```python
from build123d import *

# Parameters (mm, degrees)
SKETCH1_W           = 53
SKETCH1_H           = 53
BOSS_EXTRUDE1_DEPTH = 14.5
BOSS_EXTRUDE2_DEPTH = 53
SKETCH5_R           = 68.311173766
CUT_EXTRUDE1_DEPTH  = 60
SCALE1_SCALE        = 4


with BuildPart() as part:
    # Sketch1 → Boss-Extrude1 (new body)
    with BuildSketch(Plane(origin=(0, 0, 0), x_dir=(0, 0, -1), z_dir=(1, 0, 0))):
        with Locations((-26.5, -26.5)):
            Rectangle(SKETCH1_W, SKETCH1_H)
    extrude(amount=BOSS_EXTRUDE1_DEPTH)

    # Sketch2 → Boss-Extrude2 (add)
    with BuildSketch(Plane.XZ.offset(53)):
        Polygon((0, 53), (-15.864497794, 64.526232333), (-15.864497794, -11.526232333), (0, 0), align=None)
    extrude(amount=-BOSS_EXTRUDE2_DEPTH)

    # Sketch5 → Cut-Extrude1 (cut)
    with BuildSketch(Plane(origin=(0, 0, 0), x_dir=(1, 0, 0), z_dir=(0, 1, 0))):
        with Locations((-74.352498141, -26.670023257)):
            Circle(SKETCH5_R)
    extrude(amount=-CUT_EXTRUDE1_DEPTH, mode=Mode.SUBTRACT)


with BuildPart() as part_1:
    # Scale1: scaled about (0, 0, 0)
    add(part.part.scale(SCALE1_SCALE))


solid = part_1.part
```
Here's how the part is built. I have some questions about the finished solid (model axes, mm). A direction names the side the tool comes from. Round coordinates to 2 decimals unless told otherwise and drop trailing zeros. Write each loop counter-clockwise with the first axis right and the second up, starting at its lowest first coordinate (ties: lowest second). Pieces come first, ordered by that corner, then holes.
Q1. Please list where these lines run through material, in increasing order: probe 1 along Z at (x, y) = (53.5, -122.5); probe 2 along Z at (x, y) = (-53, -155); probe 3 along X at (y, z) = (-73.5, 75.5).
Q2. If we section it at B-B on y = -125: Write out the boundary of the cut face in (x, z), plus the area to 3 significant figures.
Q3. Will these pins go through, and if not, where does the flat tip stop? P1, Ø10, axis at y = -47.5, z = 176.5, coming from the -X side; P2, Ø4, axis at x = 22, y = -52, coming from the +Z side; P3, Ø8, axis at x = 43, y = -82.5, coming from the -Z side.
Q4. Which directions (+Z, -Z, +X, -X, +Y, -Y) give clear straight access to the entire face, cutting with the end or side of a thin tool? Please do faces 5 (the flat face through (29, -107, 0)), 6 (the flat face through (-63.458, -107, -40)).
Q5. If we section it at A-A on x = -32: Write out the boundary of the cut face in (y, z).
Q6. If we section it at C-C on x = 32.5: Write out the boundary of the cut face in (y, z).
Q7. If we mould it in two halves opening along Z, with no side actions, what happens to faces 1 (the flat face through (29, -107, 212)), 2 (the flat face through (10, 0, 108)), 3 (the flat face through (-32.173, -107.484, -23.375)), 4 (the cylindrical face through (-24.173, -104.516, 108.757))? For each: +Z half, -Z half, draft (parallel to the pull), parting line (faces both ways), or undercut.
Q8. If we section it at D-D on z = 229.5: Write out the boundary of the cut face in (x, y), plus the area to 3 significant figures.
Answer below:
1. probe 1: z = 0 to 212
1. probe 2: z = -38.51 to -15.49, 228.85 to 250.51
1. probe 3: x = -25.95 to 58
2. outline: (-63.46, -46.1) - (0, 0) - (58, 0) - (58, 212) - (0, 212) - (-63.46, 258.1) - (-63.46, 247.85) arc R273.24 cw to (-63.46, -34.49) - close
2. area: 21,200 mm2
3. P1: stops at x = -34.61
3. P2: stops at z = 212
3. P3: stops at z = 0
4. face 5: -Z, +X, +Y, -Y
4. face 6: +Z, -Z, -X, +Y, -Y
5. outline: (-212, -23.25) - (0, -23.25) - (0, 41.72) - (-212, 41.72) - close; (-212, 171.64) - (0, 171.64) - (0, 235.25) - (-212, 235.25) - close
6. outline: (-212, 0) - (0, 0) - (0, 212) - (-212, 212) - close
7. face 1: +Z half
7. face 2: draft
7. face 3: -Z half
7. face 4: undercut
8. outline: (-53.32, -212) - (-24.09, -212) - (-24.09, 0) - (-53.32, 0) - close
8. area: 6,200 mm2
